Build history of the part. All positions in model axes, mm. A direction names the side the tool comes from. Give positions to 0.01 mm unless a question says otherwise; leave off trailing zeros. Loops run counter-clockwise (first coordinate to the right, second up) from the corner with the lowest first, then second, coordinate; pieces in that order, holes last. Notation, with made-up numbers: (-19, -38) - (28, -38) arc R28 cw to (28, -5) - close; hole circle Ø10 at (12, 7.25). An arc over 180 degrees is marked (long way). Return JSON: item names as keys, results as strings. Group by question number.
1) Slice it at B-B (x = 12.5). List the corners of the cut face in (y, z), and give its area (3 significant figures).
2) 3-axis set-ups, long thin cutter, end or side, ignore diameter. For faces 1 (the face through (25, -14, 2)), 2 (the face through (-21.769, -3.793, 3.768)), 3 (the face through (23.4, 27.92, 13.91)), 4 (the face through (24, 9, 11)), 5 (the face through (-30.429, 9, 9)): which of +Z, -Z, +X, -X, +Y, -Y reach the whole face in a straight line?
3) Slice it at A-A (y = 0). List the corners of the cut face in (x, z).
4) Mould opens along Z. For faces 6 (the face through (-47.399, -17.358, 15.885)), 7 (the face through (32, 14, 10)), 8 (the face through (24.055, 28.554, 8.944)) say: released by +Z, released by -Z, zero draft, split by the parting line, or undercut.
5) Slice it at C-C (y = 36.5). List the corners of the cut face in (x, z), and give its area (3 significant figures).
6) Drop flat-ended pins along their axis: pin 1 (5.5 mm diameter, centred on x = -27, z = 1.5, fed in from -Y); pin 2 (1.6 mm diameter, centred on x = 31, z = 9, fed in from -Y); pin 3 (5 mm diameter, centred on y = 12, z = 3, fed in from -X). Give the stop position or say it passes through.
7) Drill centre lines: probe 1 along X at (y, z) = (11, 12.25); probe 2 along Z at (x, y) = (5, 29.5); probe 3 along Y at (x, z) = (24, 0.95). Where is each one in solid material? Low to high. Write a range as from..to.
```python
from build123d import *

# Parameters (mm, degrees)
SKETCH2_W                = 70
SKETCH2_H                = 28
BOSS_EXTRUDE1_DEPTH      = 5
CUT_NUT_DEPTH            = 2.5
SKETCH4_R                = 2.4
CUT_SCREW_DEPTH          = 38.7789624
SKETCH8_R                = 11
CUT_HOT_END_DEPTH        = 39.026306684
SKETCH11_W               = 22
SKETCH11_H               = 14
CUT_EXTRUDE8_DEPTH       = 39.026306684
BOSS_FAN_DEPTH           = 5
SKETCH9_R                = 2
CUT_FAN_SCREW_DEPTH      = 67.437703487
SKETCH10_R               = 18.5
CUT_EXTRUDE7_DEPTH       = 67.437703487
FILLET2_R                = 2
SKETCH12_W               = 3.5
SKETCH12_H               = 9.97245834
BOSS_BACK_HOOK_DEPTH     = 8
BOSS_BACK_HOOK_TOP_DEPTH = 9.97245834
SKETCH17_R               = 2.5
BOSS_EXTRUDE10_DEPTH     = 6
BOSS_FRONT_SUPPORT_REACH = 58.104
BOSS_FRONT_HOOK_DEPTH    = 8
SKETCH25_R               = 2.5
BOSS_FRONT_PIN_DEPTH     = 6
BOSS_FRONT_CURVE_DEPTH   = 5
CUT_EXTRUDE9_DEPTH       = 68.152189514


with BuildPart() as part:
    # Sketch2 → Boss-Extrude1 (new body)
    with BuildSketch(Plane.XY):
        Rectangle(SKETCH2_W, SKETCH2_H)
    extrude(amount=BOSS_EXTRUDE1_DEPTH)

    # Sketch3 → Cut-Nut (cut)
    with BuildSketch(Plane.XY.offset(5)):
        Polygon((28.4, 2.540341184), (24, 5.080682369), (19.6, 2.540341184), (19.6, -2.540341184), (24, -5.080682369), (28.4, -2.540341184), align=None)
    cut_nut = extrude(amount=-CUT_NUT_DEPTH, mode=Mode.SUBTRACT)

    # Sketch4 → Cut-Screw (cut, through all)
    with BuildSketch(Plane.XY.offset(2.5)):
        with Locations((24, 0)):
            Circle(SKETCH4_R)
    cut_screw = extrude(amount=-CUT_SCREW_DEPTH, mode=Mode.SUBTRACT)

    # Mirror1: Cut-Nut, Cut-Screw across plane
    add(cut_nut.mirror(Plane(origin=(0, 0, 0), x_dir=(0, 0, 1), z_dir=(1, 0, 0))), mode=Mode.SUBTRACT)
    add(cut_screw.mirror(Plane(origin=(0, 0, 0), x_dir=(0, 0, 1), z_dir=(1, 0, 0))), mode=Mode.SUBTRACT)

    # Sketch8 → Cut-Hot End (cut, through all)
    with BuildSketch(Plane.XY.offset(5)):
        Circle(SKETCH8_R)
    extrude(amount=-CUT_HOT_END_DEPTH, mode=Mode.SUBTRACT)

    # Sketch11 → Cut-Extrude8 (cut, through all)
    with BuildSketch(Plane.XY.offset(5)):
        with Locations((0, -7)):
            Rectangle(SKETCH11_W, SKETCH11_H)
    extrude(amount=-CUT_EXTRUDE8_DEPTH, mode=Mode.SUBTRACT)

    # Sketch6 → Boss-Fan (add)
    with BuildSketch(Plane(origin=(-17.5, 0, -17.5), x_dir=(-0.7071067811865488, 0, 0.7071067811865464), z_dir=(-0.7071067811865464, 0, -0.7071067811865488))):
        with BuildLine():
            Line((38.748737342, 20.5), (44.748737342, 20.5))
            Line((44.748737342, 20.5), (44.748737342, -20.5))
            Line((44.748737342, -20.5), (38.748737342, -20.5))
            add(Edge.make_bspline(
                [(24.748737342, -14), (30.971356168, -14), (32.526118515, -20.5), (38.748737342, -20.5)],
                knots=[0, 0, 0, 0, 1, 1, 1, 1], degree=3))
            Line((24.748737342, -14), (24.748737342, 14))
            add(Edge.make_bspline(
                [(24.748737342, 14), (30.971356168, 14), (32.526118515, 20.5), (38.748737342, 20.5)],
                knots=[0, 0, 0, 0, 1, 1, 1, 1], degree=3))
        make_face()
    extrude(amount=-BOSS_FAN_DEPTH)

    # Sketch9 → Cut-Fan Screw (cut, through all)
    with BuildSketch(Plane(origin=(-17.5, 0, -17.5), x_dir=(-0.7071067811865487, 1.3344026738283447e-14, 0.7071067811865464), z_dir=(-0.7071067811865464, 1.3877787807814728e-14, -0.7071067811865487))):
        with Locations((38.748737342, 16.5)):
            Circle(SKETCH9_R)
    cut_fan_screw = extrude(amount=-CUT_FAN_SCREW_DEPTH, mode=Mode.SUBTRACT)

    # Mirror-Fan Screw: Cut-Fan Screw across plane
    add(cut_fan_screw.mirror(Plane.ZX), mode=Mode.SUBTRACT)

    # Sketch10 → Cut-Extrude7 (cut, through all)
    with BuildSketch(Plane(origin=(-17.5, 0, -17.5), x_dir=(-0.7071067811865488, 1.4278108609963275e-14, 0.7071067811865464), z_dir=(-0.7071067811865464, 1.3877787807814742e-14, -0.7071067811865488))):
        with Locations((55.248737342, 0)):
            Circle(SKETCH10_R)
    extrude(amount=-CUT_EXTRUDE7_DEPTH, mode=Mode.SUBTRACT)

    # Fillet2
    fillet2_edges = [part.edges().sort_by_distance(p)[0] for p in [
        (-47.374368671, -15.231546212, 15.909902577),
        (-47.374368671, 15.231546212, 15.909902577),
        (-47.374368671, 20.5, 15.909902577),
        (-47.374368671, -20.5, 15.909902577),
    ]]
    fillet(fillet2_edges, radius=FILLET2_R)

    # Sketch12 → Boss-Back Hook (add)
    with BuildSketch(Plane.XY.offset(5)):
        with Locations((-32.178932188, 9.01377083)):
            Rectangle(SKETCH12_W, SKETCH12_H)
    boss_back_hook = extrude(amount=BOSS_BACK_HOOK_DEPTH)

    # Sketch14 → Boss-Back Hook Top (add)
    with BuildSketch(Plane.XZ.offset(-4.02754166)):
        Polygon((-30.428932188, 13), (-28.428932188, 15), (-29.428932188, 16), (-30.928932188, 16), (-33.928932188, 13), align=None)
    boss_back_hook_top = extrude(amount=-BOSS_BACK_HOOK_TOP_DEPTH)

    # Mirror-Back Hook: Boss-Back Hook, Boss-Back Hook Top across plane
    add(boss_back_hook.mirror(Plane(origin=(0, 0, 0), x_dir=(0, 0, 1), z_dir=(1, 0, 0))))
    add(boss_back_hook_top.mirror(Plane(origin=(0, 0, 0), x_dir=(0, 0, 1), z_dir=(1, 0, 0))))

    # Sketch17 → Boss-Extrude10 (add)
    with BuildSketch(Plane.XY.offset(5)):
        with Locations(Location((-24, 9.01377083, 0), (0, 0, 180))):
            Circle(SKETCH17_R)
        with Locations(Location((24, 9.01377083, 0), (0, 0, 180))):
            Circle(SKETCH17_R)
    extrude(amount=BOSS_EXTRUDE10_DEPTH)

    # Boss-Front Support: up to this face of the body (flat: up to its plane)
    boss_front_support_end = Plane(part.part.faces().sort_by_distance((23, -13.265266046, 5))[0])
    # Sketch20 → Boss-Front Support (add, up to the picked face)
    with BuildSketch(Plane(origin=(0, 0, 0), x_dir=(-1, 0, 0), z_dir=(0, 0, -1)), mode=Mode.PRIVATE) as boss_front_support_sk1:
        with BuildLine():
            Line((24.083189158, 33), (15.583240043, 24.529411765))
            ThreePointArc((15.583240043, 24.529411765), (19.23814858, 19.67209629), (21.424285286, 14))
            Line((21.424285286, 14), (33.630343442, 14))
            ThreePointArc((33.630343442, 14), (30.380305483, 24.265550718), (24.083189158, 33))
        make_face()
    boss_front_support_tool1 = split(extrude(boss_front_support_sk1.sketch, amount=-BOSS_FRONT_SUPPORT_REACH, mode=Mode.PRIVATE), bisect_by=boss_front_support_end, keep=Keep.BOTH, mode=Mode.PRIVATE)
    boss_front_support = boss_front_support_tool1.solids().sort_by(Axis((-24.942204, 21.980876, 0), (0, 0, 1)))[0]
    add(boss_front_support)

    # Sketch21 → Boss-Front Hook (add)
    with BuildSketch(Plane.XY.offset(5)):
        with BuildLine():
            Line((-24.416846712, 32.660464844), (-22.262419061, 30.57277677))
            ThreePointArc((-22.262419061, 30.57277677), (-24.079068363, 28.524304515), (-25.707884563, 26.323529412))
            Line((-25.707884563, 26.323529412), (-28.19574436, 28))
            ThreePointArc((-28.19574436, 28), (-26.409300785, 30.413753339), (-24.416846712, 32.660464844))
        make_face()
    boss_front_hook = extrude(amount=BOSS_FRONT_HOOK_DEPTH)

    # Sweep-Front Hook Top: sweep along a curve in space
    with BuildLine() as sweep_front_hook_top_path:
        ThreePointArc((-25.707884563, 26.323529412, 13), (-24.079068363, 28.524304515, 13), (-22.262419061, 30.57277677, 13))
    # Sketch22 → Sweep-Front Hook Top (sweep)
    with BuildSketch(Plane(origin=(4.752413936, 4.394805718, 0), x_dir=(0, 0, -1), z_dir=(0.6958960248359726, 0.7181425503460238, 0))):
        Polygon((-13, 37.617647059), (-13, 40.617647059), (-15.611662163, 38.005984896), (-15.611662163, 36.747093005), (-14.741108108, 35.87653895), align=None)
    sweep(path=sweep_front_hook_top_path.line)

    # Sketch25 → Boss-Front Pin (add)
    with BuildSketch(Plane.XY.offset(5)):
        with Locations(Location((-19.93223769, 25.111248957, 0), (0, 0, 180))):
            Circle(SKETCH25_R)
    boss_front_pin = extrude(amount=BOSS_FRONT_PIN_DEPTH)

    # Sketch23 → Boss-Front Curve (add)
    with BuildSketch(Plane(origin=(0, 0, 0), x_dir=(-1, 0, 0), z_dir=(0, 0, -1))):
        with BuildLine():
            Line((0, 42.213351454), (0, 14))
            Line((0, 14), (33.630343442, 14))
            Line((33.630343442, 14), (24.083189158, 33))
            ThreePointArc((24.083189158, 33), (12.892690226, 39.831392494), (0, 42.213351454))
        make_face()
    boss_front_curve = extrude(amount=-BOSS_FRONT_CURVE_DEPTH)

    # Mirror5: Boss-Front Support, Boss-Front Hook, Boss-Front Pin, Boss-Front Curve across plane
    add(boss_front_support.mirror(Plane(origin=(0, 0, 0), x_dir=(0, 0, 1), z_dir=(1, 0, 0))))
    add(boss_front_hook.mirror(Plane(origin=(0, 0, 0), x_dir=(0, 0, 1), z_dir=(1, 0, 0))))
    add(boss_front_pin.mirror(Plane(origin=(0, 0, 0), x_dir=(0, 0, 1), z_dir=(1, 0, 0))))
    add(boss_front_curve.mirror(Plane(origin=(0, 0, 0), x_dir=(0, 0, 1), z_dir=(1, 0, 0))))

    # Sweep2: sweep along a curve in space
    with BuildLine() as sweep2_path:
        ThreePointArc((25.707884563, 26.323529412, 13), (24.079068363, 28.524304515, 13), (22.262419061, 30.57277677, 13))
    # Sketch24 → Sweep2 (sweep)
    with BuildSketch(Plane(origin=(-4.170823776, 6.189446367, 0), x_dir=(0.8292865988159824, 0.5588235294117634, 0), z_dir=(0.5588235294117634, -0.8292865988159824, 0))):
        Polygon((36.029411765, 13), (39.029411765, 13), (36.273559232, 15.755852533), (35.110794254, 15.755852533), (34.192176743, 14.837235022), align=None)
    sweep(path=sweep2_path.line)

    # Sketch26 → Cut-Extrude9 (cut, through all)
    with BuildSketch(Plane(origin=(0, 0, 0), x_dir=(-1, 0, 0), z_dir=(0, 0, -1))):
        with BuildLine():
            Line((-16, -14), (-16, 14.213351454))
            ThreePointArc((-16, 14.213351454), (0, 30.213351454), (16, 14.213351454))
            Line((16, 14.213351454), (16, -14))
            Line((16, -14), (-16, -14))
        make_face()
    extrude(amount=-CUT_EXTRUDE9_DEPTH, mode=Mode.SUBTRACT)


solid = part.part
```
Results:
{
 "1": {"outline": "(24.2, 0) - (39.98, 0) - (39.98, 5) - (24.2, 5) - close", "area": "78.9 mm2"},
 "2": {"face 1": "+Z, -Z, +X, -Y", "face 2": "+Z", "face 3": "-Y", "face 4": "+Z, -Y", "face 5": "+Y, -Y"},
 "3": {"outline": "(-43.49, 8.49) - (-35, 0) - (-26.4, 0) - (-26.4, 2.5) - (-28.4, 2.5) - (-28.4, 5) - (-32.93, 5) - (-39.95, 12.02) - close; (-21.6, 0) - (-16, 0) - (-16, 5) - (-19.6, 5) - (-19.6, 2.5) - (-21.6, 2.5) - close; (16, 0) - (21.6, 0) - (21.6, 2.5) - (19.6, 2.5) - (19.6, 5) - (16, 5) - close; (26.4, 0) - (35, 0) - (35, 5) - (28.4, 5) - (28.4, 2.5) - (26.4, 2.5) - close"},
 "4": {"face 6": "released by +Z", "face 7": "zero draft", "face 8": "undercut"},
 "5": {"outline": "(-19.48, 0) - (19.48, 0) - (19.48, 5) - (-19.48, 5) - close", "area": "195 mm2"},
 "6": {"pin 1": "y = -14", "pin 2": "y = 4.03", "pin 3": "x = -40.5"},
 "7": {"probe 1": "-44.85..-40.18, -33.93..-30.43, 30.43..33.93", "probe 2": "0..5", "probe 3": "-14..-2.4, 2.4..33.07"}
}
